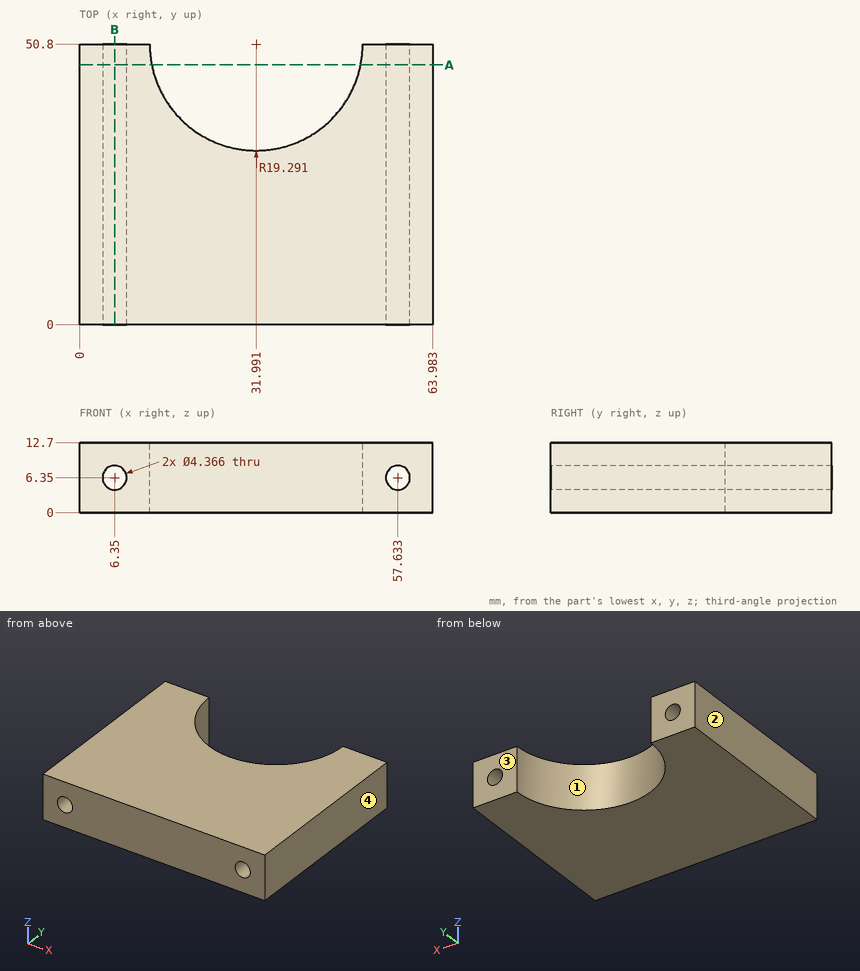
Here's the drawing with two shaded views (mm, measured from the low corner). I have some questions. Give positions to 0.01 mm unless a question says otherwise; leave off trailing zeros. Order: outer loops, then holes, each group sorted by start corner. A loop starts at its lowest first (then second) coordinate and runs counter-clockwise, first axis right, second up.
Q1. We'd pull the mould along X, two halves only. Please class the marked faces 1, 2, 3 and 4: +X half, -X half, draft (parallel to the pull), parting line (faces both ways), or undercut.
Q2. Suppose I cut it at B-B, the plane x = 6.35. Write out the boundary of the cut face in (y, z).
Q3. If I drill on line 1 along X through (y, z) = (28.5, 6.75) (1 decimal); line 2 along Z through (x, y) = (6.35, 34); line 3 along X through (y, z) = (15, 8.25) (1 decimal), over which ranges is the centre line in solid material (lowest first)?
Q4. Suppose I cut it at A-A, the plane y = 47. Count the separate pieces of the cut face and the enclosed holes in it, and give its area (3 significant figures).
Q5. I'm going to push flat-ended pins straight in: P1, Ø1.5, axis at y = 10, z = 8, coming from the -X side; P2, Ø3, axis at x = 36, z = 3.5, coming from the +Y side; P3, Ø6, axis at x = 44, z = 3, coming from the +Y side. Where does each tip first touch, or does it pass through?
Solution:
1. face 1: undercut
1. face 2: -X half
1. face 3: draft
1. face 4: +X half
2. outline: (0, 0) - (50.8, 0) - (50.8, 4.17) - (0, 4.17) - close; (0, 8.53) - (50.8, 8.53) - (50.8, 12.7) - (0, 12.7) - close
3. line 1: x = 0 to 4.2, 8.5 to 55.5, 59.8 to 64
3. line 2: z = 0 to 4.17, 8.53 to 12.7
3. line 3: x = 0 to 5.3, 7.4 to 56.6, 58.7 to 64
4. separate pieces: 2
4. enclosed holes: 2
4. area: 302 mm2
5. P1: stops at x = 0
5. P2: stops at y = 32.31
5. P3: stops at y = 38.68
